Read the model definition and answer for the solid it produces. Units are mm, in the model's axes. Give positions to 0.01 mm unless a question says otherwise; leave off trailing zeros. Order: outer loops, then holes, each group sorted by start corner. A loop starts at its lowest first (then second) coordinate and runs counter-clockwise, first axis right, second up. Notation, with made-up numbers: M 58.25,16 L 82.25,16 A25 ccw 82.25,51 Z; hole C 14.5,16 d1. An arc over 180 degrees is marked long. One line per item, written item: value.
from build123d import *

# Parameters (mm, degrees)
BOSS_EXTRUDE1_DEPTH = 3.175
SKETCH2_R           = 2
CUT_EXTRUDE1_DEPTH  = 3.175
SKETCH3_R           = 3
CUT_EXTRUDE2_DEPTH  = 5.08


with BuildPart() as part:
    # Sketch1 → Boss-Extrude1 (new body)
    with BuildSketch(Plane.XY):
        Polygon((0, 0), (0, 228.6), (177.8, 228.6), (177.8, 0), (140.97, 0), (140.97, 107.188), (36.83, 107.188), (36.83, 0), align=None)
    extrude(amount=BOSS_EXTRUDE1_DEPTH)

    # Sketch2 → Cut-Extrude1 (cut)
    with BuildSketch(Plane(origin=(0, 0, 0), x_dir=(-1, 0, 0), z_dir=(0, 0, -1))):
        with Locations((-22.86, 111.071616712)):
            Circle(SKETCH2_R)
        with Locations((-5.080886425, 111.071616712)):
            Circle(SKETCH2_R)
        with Locations((-22.86, 75.511616712)):
            Circle(SKETCH2_R)
        with Locations((-5.080886425, 75.334076645)):
            Circle(SKETCH2_R)
    extrude(amount=-CUT_EXTRUDE1_DEPTH, mode=Mode.SUBTRACT)

    # Sketch3 → Cut-Extrude2 (cut)
    with BuildSketch(Plane(origin=(0, 0, 0), x_dir=(-1, 0, 0), z_dir=(0, 0, -1))):
        with Locations((-151.12245979, 123.444)):
            Circle(SKETCH3_R)
        with Locations((-151.12245979, 87.884)):
            Circle(SKETCH3_R)
    extrude(amount=-CUT_EXTRUDE2_DEPTH, mode=Mode.SUBTRACT)


solid = part.part
1) Find section A-A, the plane y = 100. Write down the section's boundary in (x, z) (3 decimals).
Reported:
outline: M 0,0 L 36.83,0 L 36.83,3.175 L 0,3.175 Z; M 140.97,0 L 177.8,0 L 177.8,3.175 L 140.97,3.175 Z
2) Consider probe 1 along X at (y, z) = (25.5, 1.1); probe 2 along Y at (x, z) = (22.86, 2.45); probe 3 along Y at (x, z) = (89.5, 1.45). Determine where each line is inside the solid, lowest interval first.
Reported:
probe 1: x = 0 to 36.83, 140.97 to 177.8
probe 2: y = 0 to 73.51, 77.51 to 109.07, 113.07 to 228.6
probe 3: y = 107.19 to 228.6
3) Find section C-C, the plane x = 110. Write down the section's boundary in (y, z) (3 decimals), plus the area to 3 significant figures.
Reported:
outline: M 107.188,0 L 228.6,0 L 228.6,3.175 L 107.188,3.175 Z
area: 385 mm^2
4) Find section B-B, the plane z = 0.6. Write down the section's boundary in (x, y).
Reported:
outline: M 0,0 L 36.83,0 L 36.83,107.19 L 140.97,107.19 L 140.97,0 L 177.8,0 L 177.8,228.6 L 0,228.6 Z; hole C 5.08,75.33 d4; hole C 5.08,111.07 d4; hole C 22.86,75.51 d4; hole C 22.86,111.07 d4; hole C 151.12,87.88 d6; hole C 151.12,123.44 d6
5) Each of these flat-tipped pins is pushed along its axis until it touches: pin 1 Ø1 at (x, z) = (83, 2) entering from -Y; pin 2 Ø3 at (x, y) = (22.86, 111.07) entering from -Z. Where does it stop, or does it pass through?
Reported:
pin 1: stops at y = 107.19
pin 2: passes through
6) Determine the mould class of faces 1 (the face through (90, 141, 3.175)), 2 (the face through (148.261, 124.345, 1.565)) for opening direction Y: +Y half, -Y half, draft (parallel to the pull), parting line (faces both ways), or undercut.
Reported:
face 1: draft
face 2: undercut
